from build123d import *

# Parameters (mm, degrees)
SKETCH036_R             = 2.25
PAD016_DEPTH            = 2.25
SKETCH037_W             = 11
SKETCH037_H             = 1
PAD017_DEPTH            = 10
SKETCH038_W             = 15.25
SKETCH038_H             = 9.5
PAD018_DEPTH            = 17.25
SKETCH039_W             = 11.75
SKETCH039_H             = 15.75
POCKET007008_DEPTH      = 9.501
SKETCH040_R             = 1
POCKET007009_DEPTH      = 23.501
PAD019_DEPTH            = 5
SKETCH043_W             = 1
SKETCH043_H             = 7
POCKET007011_DEPTH      = 3
BODY008_PLACEMENT_ANGLE = 90


with BuildPart() as part:
    # Sketch036 → Pad016 (new body)
    with BuildSketch(Plane.XY):
        Polygon((-75.5, -11), (-68, -11), (-68, -22.5), (-52, -22.5), (-52, -32), (-75.5, -32), align=None)
        with Locations((-72, -16)):
            Circle(SKETCH036_R, mode=Mode.SUBTRACT)
        with Locations((-72, -28)):
            Circle(SKETCH036_R, mode=Mode.SUBTRACT)
        with Locations((-57, -28)):
            Circle(SKETCH036_R, mode=Mode.SUBTRACT)
    extrude(amount=PAD016_DEPTH)

    # Sketch037 (on DatumPlane) → Pad017 (join)
    with BuildSketch(Plane(origin=(-68, -22.5, 0), x_dir=(1, 0, 0), z_dir=(0, -1, 0))):
        with Locations((8.5, 1.75)):
            Rectangle(SKETCH037_W, SKETCH037_H)
    extrude(amount=-PAD017_DEPTH)

    # Sketch038 (on DatumPlane) → Pad018 (join)
    with BuildSketch(Plane.XY.offset(2.25)):
        with Locations((-59.625, -27.25)):
            Rectangle(SKETCH038_W, SKETCH038_H)
    extrude(amount=PAD018_DEPTH)

    # Sketch039 (on DatumPlane) → Pocket007008 (cut, through all)
    with BuildSketch(Plane(origin=(-68, -22.5, 0), x_dir=(1, 0, 0), z_dir=(0, -1, 0))):
        with Locations((8.125, 10.125)):
            Rectangle(SKETCH039_W, SKETCH039_H)
    extrude(amount=POCKET007008_DEPTH, mode=Mode.SUBTRACT)

    # Sketch040 (on DatumPlane) → Pocket007009 (cut, through all)
    with BuildSketch(Plane(origin=(-52, -27.25, 2.25), x_dir=(0, -1, 0), z_dir=(-1, 0, 0))):
        with Locations((0, 8.625)):
            Circle(SKETCH040_R)
    extrude(amount=POCKET007009_DEPTH, mode=Mode.SUBTRACT)

    # Sketch042 (on DatumPlane) → Pad019 (join)
    with BuildSketch(Plane(origin=(-68, -22.5, 0), x_dir=(1, 0, 0), z_dir=(0, -1, 0))):
        Polygon((14.5, 18.5), (14.5, 2.25), (14, 2.25), (14, 18), (2.25, 18), (2.25, 2.25), (1.75, 2.25), (1.75, 18.5), align=None)
    extrude(amount=-PAD019_DEPTH)

    # Sketch043 (on DatumPlane) → Pocket007011 (cut)
    with BuildSketch(Plane(origin=(-68, -17.5, 0), x_dir=(-1, 0, 0), z_dir=(0, 1, 0))):
        with Locations((-14, 15)):
            Rectangle(SKETCH043_W, SKETCH043_H)
    extrude(amount=-POCKET007011_DEPTH, mode=Mode.SUBTRACT)


with BuildPart() as part_1:
    # Body002 placement: moved
    add(part.part.moved(Location((0, 0, 22))))


with BuildPart() as part_2:
    # Body008 placement: moved
    add(part_1.part.moved(Location((24, 10, 52))).rotate(Axis((24, 10, 52), (1, 0, 0)), BODY008_PLACEMENT_ANGLE))


solid = part_2.part
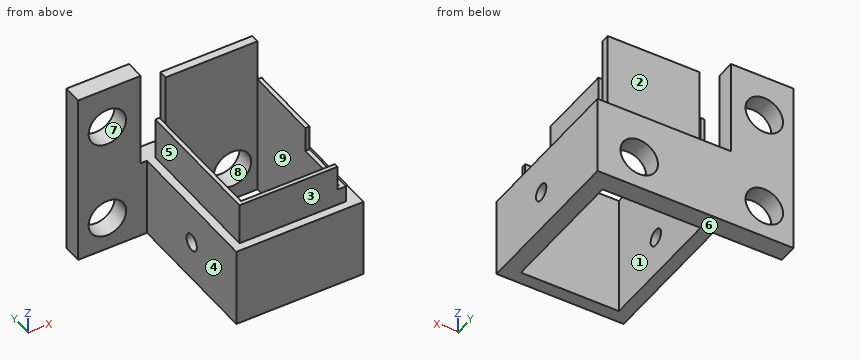
CAD build for the part. Positions are in the model's coordinates, mm. Face numbers are marked on the shaded views. A direction names the side the tool comes from. Round coordinates to 2 decimals unless told otherwise and drop trailing zeros. Loops run counter-clockwise (first coordinate to the right, second up) from the corner with the lowest first, then second, coordinate; pieces in that order, holes last. Notation, with made-up numbers: (65.25, -7) - (74.25, -7) arc R23 cw to (74.25, 31) - close; hole circle Ø4 at (56, -31). An arc over 180 degrees is marked (long way). Put each result on its own line as item: value.
1. Slice it at C-C on y = -16. List the corners of the cut face in (x, z).
Geometry check:
outline: (-43.25, 20) - (-41.75, 20) - (-41.75, 34.5) - (-42.25, 34.5) - (-42.25, 29.5) - (-43.25, 29.5) - close; (-30, 20) - (-28, 20) - (-28, 29.5) - (-29.5, 29.5) - (-29.5, 34.5) - (-30, 34.5) - close
2. Pin check, flat tips, straight feed: P1, Ø3, axis at y = -22.875, z = 24.75, coming from the -X side; P2, Ø5, axis at x = -48, z = 24, coming from the -Y side; P3, Ø1.5, axis at x = -33, z = 24, coming from the +Y side. Stop position of each tip, or through.
Geometry check:
P1: x = -43.25
P2: y = -14.25
P3: y = -30
3. 3-axis set-ups, long thin cutter, end or side, ignore diameter. For the marked faces 1, 2, 3, 4 and 5: which of +Z, -Z, +X, -X, +Y, -Y reach the whole face in a straight line?
Geometry check:
face 1: +Z, -Z
face 2: +Z, +X, +Y
face 3: +Z, +X, -X, -Y
face 4: +Z, -Z, -X, -Y
face 5: +Z, -X, +Y, -Y
4. Slice it at A-A on x = -33. List the corners of the cut face in (y, z).
Geometry check:
outline: (-31.5, 20) - (-30, 20) - (-30, 34.5) - (-30.5, 34.5) - (-30.5, 29.5) - (-31.5, 29.5) - close; (-14.25, 20) - (-12, 20) - (-12, 21.75) - (-14.25, 21.75) - close; (-14.25, 26.25) - (-12, 26.25) - (-12, 29.5) - (-13.25, 29.5) - (-13.25, 39.5) - (-14.25, 39.5) - close
5. Slice it at D-D on z = 24.75. List the corners of the cut face in (x, y) (3 decimals), and give its area (3 significant figures).
Geometry check:
outline: (-51.5, -14.25) - (-50.121, -14.25) - (-50.121, -12) - (-51.5, -12) - close; (-45.879, -14.25) - (-43.25, -14.25) - (-43.25, -21.875) - (-41.75, -21.875) - (-41.75, -14.25) - (-35.121, -14.25) - (-35.121, -12) - (-45.879, -12) - close; (-43.25, -31.5) - (-28, -31.5) - (-28, -23.875) - (-30, -23.875) - (-30, -30) - (-41.75, -30) - (-41.75, -23.875) - (-43.25, -23.875) - close; (-30.879, -14.25) - (-30, -14.25) - (-30, -21.875) - (-28, -21.875) - (-28, -12) - (-30.879, -12) - close
area: 105 mm²
6. Two-plate mould, pull along Z, no slides. Class the marked faces 6, 7, 8 and 9: released by +Z, released by -Z, zero draft, split by the parting line, or undercut.
Geometry check:
face 6: released by -Z
face 7: undercut
face 8: undercut
face 9: zero draft
7. Wall check: line 1 (Z direction, x = -48, y = -13.2); line 2 (X direction, y = -24, z = 21.25); line 3 (Y direction, x = -29.15, z = 24.75) (3 decimals). Give the ranges that are in metal, low to high.
Geometry check:
line 1: 20 to 21.75, 26.25 to 33.75, 38.25 to 41
line 2: -43.25 to -41.75, -30 to -28
line 3: -31.5 to -23.875, -21.875 to -12
8. Slice it at B-B on z = 36. List the corners of the cut face in (x, y).
Geometry check:
outline: (-51.5, -14.25) - (-50.25, -14.25) - (-50.25, -12) - (-51.5, -12) - close; (-45.75, -14.25) - (-44, -14.25) - (-44, -12) - (-45.75, -12) - close; (-41, -14.25) - (-30, -14.25) - (-30, -13.25) - (-41, -13.25) - close
